from build123d import *

# Parameters (mm, degrees)
SKETCH2_R            = 3.9
BOSS_EXTRUDE1_DEPTH  = 12
SKETCH3_R            = 6
BOSS_EXTRUDE2_DEPTH  = 2
BOSS_EXTRUDE3_START  = 2
SKETCH4_R            = 6
BOSS_EXTRUDE3_DEPTH  = 2
SKETCH5_W            = 19.497175456
SKETCH5_H            = 13.883202756
CUT_EXTRUDE1_DEPTH   = 5
SKETCH6_W            = 2
SKETCH6_H            = 6.63324958
BOSS_EXTRUDE4_DEPTH  = 8
SKETCH7_W            = 16
SKETCH7_H            = 10
BOSS_EXTRUDE5_DEPTH  = 3
SKETCH8_R            = 12.5
BOSS_EXTRUDE6_DEPTH  = 40
SKETCH10_R           = 2.1
CUT_EXTRUDE2_DEPTH   = 21
BOSS_EXTRUDE7_DEPTH  = 12
FILLET1_R            = 0.5
SKETCH11_W           = 2
SKETCH11_H           = 19
BOSS_EXTRUDE8_DEPTH  = 11.3
SKETCH13_W           = 2
SKETCH13_H           = 19
BOSS_EXTRUDE9_DEPTH  = 11.3
SKETCH14_W           = 16
SKETCH14_H           = 19
BOSS_EXTRUDE10_DEPTH = 1
SKETCH15_W           = 16
SKETCH15_H           = 19
BOSS_EXTRUDE11_DEPTH = 1
SKETCH16_W           = 16
SKETCH16_H           = 7.233308129
CUT_EXTRUDE3_DEPTH   = 7
SKETCH17_W           = 16
SKETCH17_H           = 7.233308129
CUT_EXTRUDE4_DEPTH   = 7
SKETCH18_W           = 2
SKETCH18_H           = 1
BOSS_EXTRUDE12_DEPTH = 6.633249581
SKETCH19_W           = 2
SKETCH19_H           = 1
BOSS_EXTRUDE13_DEPTH = 6.633249581


with BuildPart() as part:
    # Sketch2 → Boss-Extrude1 (new body)
    with BuildSketch(Plane(origin=(0, 0, 0), x_dir=(0, 0, -1), z_dir=(1, 0, 0))):
        Circle(SKETCH2_R)
    extrude(amount=BOSS_EXTRUDE1_DEPTH)

    # Sketch3 → Boss-Extrude2 (add)
    with BuildSketch(Plane(origin=(12, 0, 0), x_dir=(0, 0, -1), z_dir=(1, 0, 0))):
        Circle(SKETCH3_R)
    extrude(amount=BOSS_EXTRUDE2_DEPTH)

    # Sketch4 → Boss-Extrude3 (add)
    with BuildSketch(Plane.ZY.offset(BOSS_EXTRUDE3_START)):
        with Locations(Location((0, 0, 0), (0, 0, 180))):
            Circle(SKETCH4_R)
    extrude(amount=-BOSS_EXTRUDE3_DEPTH)

    # Sketch5 → Cut-Extrude1 (cut)
    with BuildSketch(Plane(origin=(0, 5, 0), x_dir=(1, 0, 0), z_dir=(0, 1, 0))):
        with Locations((6.056898372, 0.369839418)):
            Rectangle(SKETCH5_W, SKETCH5_H)
    extrude(amount=CUT_EXTRUDE1_DEPTH, mode=Mode.SUBTRACT)

    # Sketch6 → Boss-Extrude4 (add)
    with BuildSketch(Plane(origin=(0, 5, 0), x_dir=(1, 0, 0), z_dir=(0, 1, 0))):
        with Locations((13, 0)):
            Rectangle(SKETCH6_W, SKETCH6_H)
        with Locations((-1, 0)):
            Rectangle(SKETCH6_W, SKETCH6_H)
    extrude(amount=BOSS_EXTRUDE4_DEPTH)

    # Sketch7 → Boss-Extrude5 (add)
    with BuildSketch(Plane(origin=(0, 13, 0), x_dir=(1, 0, 0), z_dir=(0, 1, 0))):
        with Locations((6, 0)):
            Rectangle(SKETCH7_W, SKETCH7_H)
    extrude(amount=BOSS_EXTRUDE5_DEPTH)

    # Sketch8 → Boss-Extrude6 (add)
    with BuildSketch(Plane(origin=(0, 16, 0), x_dir=(1, 0, 0), z_dir=(0, 1, 0))):
        with Locations(Location((6, 0, 0), (0, 0, 270))):
            Circle(SKETCH8_R)
    extrude(amount=BOSS_EXTRUDE6_DEPTH)

    # Sketch10 → Cut-Extrude2 (cut)
    with BuildSketch(Plane(origin=(0, 56, 0), x_dir=(1, 0, 0), z_dir=(0, 1, 0))):
        with Locations(Location((6, 0, 0), (0, 0, 270))):
            Circle(SKETCH10_R)
    extrude(amount=-CUT_EXTRUDE2_DEPTH, mode=Mode.SUBTRACT)

    # Sketch12 → Boss-Extrude7 (add)
    with BuildSketch(Plane.ZY.offset(-12)):
        Polygon((-3.2, 4.2), (3.2, 4.2), (5, 9.2), (5.36, 10.2), (-5.36, 10.2), (-5, 9.2), align=None)
    extrude(amount=BOSS_EXTRUDE7_DEPTH)

    # Fillet1
    fillet1_edges = [part.edges().sort_by_distance(p)[0] for p in [
        (6, 4.2, -3.2),
        (6, 4.2, 3.2),
        (6, 10.2, 5.36),
        (6, 10.2, -5.36),
    ]]
    fillet(fillet1_edges, radius=FILLET1_R)

    # Sketch11 → Boss-Extrude8 (add)
    with BuildSketch(Plane.XY.offset(3.31662479)):
        with Locations((13, 3.5)):
            Rectangle(SKETCH11_W, SKETCH11_H)
        with Locations((-1, 3.5)):
            Rectangle(SKETCH11_W, SKETCH11_H)
    extrude(amount=BOSS_EXTRUDE8_DEPTH)

    # Sketch13 → Boss-Extrude9 (add)
    with BuildSketch(Plane(origin=(0, 0, -3.31662479), x_dir=(-1, 0, 0), z_dir=(0, 0, -1))):
        with Locations((-13, 3.5)):
            Rectangle(SKETCH13_W, SKETCH13_H)
        with Locations((1, 3.5)):
            Rectangle(SKETCH13_W, SKETCH13_H)
    extrude(amount=BOSS_EXTRUDE9_DEPTH)

    # Sketch14 → Boss-Extrude10 (add)
    with BuildSketch(Plane.XY.offset(14.61662479)):
        with Locations((6, 3.5)):
            Rectangle(SKETCH14_W, SKETCH14_H)
    extrude(amount=BOSS_EXTRUDE10_DEPTH)

    # Sketch15 → Boss-Extrude11 (add)
    with BuildSketch(Plane(origin=(0, 0, -14.61662479), x_dir=(-1, 0, 0), z_dir=(0, 0, -1))):
        with Locations((-6, 3.5)):
            Rectangle(SKETCH15_W, SKETCH15_H)
    extrude(amount=BOSS_EXTRUDE11_DEPTH)

    # Sketch16 → Cut-Extrude3 (cut)
    with BuildSketch(Plane(origin=(0, 0, -15.61662479), x_dir=(-1, 0, 0), z_dir=(0, 0, -1))):
        with Locations((-6, 9.383345935)):
            Rectangle(SKETCH16_W, SKETCH16_H)
    extrude(amount=-CUT_EXTRUDE3_DEPTH, mode=Mode.SUBTRACT)

    # Sketch17 → Cut-Extrude4 (cut)
    with BuildSketch(Plane.XY.offset(15.61662479)):
        with Locations((6, 9.383345935)):
            Rectangle(SKETCH17_W, SKETCH17_H)
    extrude(amount=-CUT_EXTRUDE4_DEPTH, mode=Mode.SUBTRACT)

    # Sketch18 → Boss-Extrude12 (add)
    with BuildSketch(Plane(origin=(0, 0, 3.31662479), x_dir=(-1, 0, 0), z_dir=(0, 0, -1))):
        with Locations((-13, -5.5)):
            Rectangle(SKETCH18_W, SKETCH18_H)
    extrude(amount=BOSS_EXTRUDE12_DEPTH)

    # Sketch19 → Boss-Extrude13 (add)
    with BuildSketch(Plane(origin=(0, 0, 3.31662479), x_dir=(-1, 0, 0), z_dir=(0, 0, -1))):
        with Locations((1, -5.5)):
            Rectangle(SKETCH19_W, SKETCH19_H)
    extrude(amount=BOSS_EXTRUDE13_DEPTH)


solid = part.part
CAD build for the part. Positions are in the model's coordinates, mm. A direction names the side the tool comes from. Coordinates: 2 decimals unless noted, no trailing zeros. Order: outer loops, then holes, each group sorted by start corner. A loop starts at its lowest first (then second) coordinate and runs counter-clockwise, first axis right, second up. Notation, with made-up numbers: (85.25, -26.75) -> (136.25, -26.75) arc R16 cw to (136.25, -16.75) -> close; hole circle Ø10 at (87, 88). An arc over 180 degrees is marked (long way). Answer in a Markdown table with one row per item.
1) Drill centre lines: line 1 (X direction, y = 51.25, z = 0); line 2 (X direction, y = 12, z = -5); line 3 (Y direction, x = 10.5, z = 10). Where is each one in solid material? Low to high.
Check values:
| item | result |
|---|---|
| line 1 | -6.5 to 3.9, 8.1 to 18.5 |
| line 2 | -2 to 0, 12 to 14 |
| line 3 | 16 to 56 |
2) Which spindle directions (+Z, -Z, +X, -X, +Y, -Y) get a long thin tool onto all of the face, cutting with end or side? Do faces 4 (the face through (6, 14, -5)), 5 (the face through (6, 14, 5)), 6 (the face through (8.082, 45.647, -0.273)), 7 (the face through (6.08, 7, 4.21)). Say none if no direction does.
Check values:
| item | result |
|---|---|
| face 4 | -Z, +X, -X |
| face 5 | +Z, +X, -X |
| face 6 | +Y |
| face 7 | none |
3) Band-saw the part on D-D (z = 0). List the corners of the cut face in (x, y).
Check values:
| item | result |
|---|---|
| outline | (-6.5, 16) -> (-2, 16) -> (-2, -6) -> (0, -6) -> (0, -3.9) -> (12, -3.9) -> (12, -6) -> (14, -6) -> (14, 16) -> (18.5, 16) -> (18.5, 56) -> (8.1, 56) -> (8.1, 35) -> (3.9, 35) -> (3.9, 56) -> (-6.5, 56) -> close; hole (0, 3.9) -> (12, 3.9) -> (12, 4.2) -> (0, 4.2) -> close; hole (0, 10.2) -> (12, 10.2) -> (12, 13) -> (0, 13) -> close |
4) Flat gauge pins, fed straight in: P1, Ø6.5, axis at y = 3, z = 4, coming from the -X side; P2, Ø8, axis at y = 42, z = -6, coming from the -X side; P3, Ø8, axis at y = 49.5, z = -5, coming from the -X side. Where does each tip first touch, or does it go through?
Check values:
| item | result |
|---|---|
| P1 | x = -2 |
| P2 | x = -6.34 |
| P3 | x = -6.46 |
5) Band-saw the part on A-A (z = 10). List the corners of the cut face in (x, y), and give its area (3 significant figures).
Check values:
| item | result |
|---|---|
| outline | (-2, -6) -> (0, -6) -> (0, 5.77) -> (-2, 5.77) -> close; (-1.5, 16) -> (13.5, 16) -> (13.5, 56) -> (-1.5, 56) -> close; (12, -6) -> (14, -6) -> (14, 5.77) -> (12, 5.77) -> close |
| area | 647 mm2 |
6) Band-saw the part on B-B (x = 6). Give the number of separate pieces and of enclosed holes in the cut face, and give its area (3 significant figures).
Check values:
| item | result |
|---|---|
| separate pieces | 5 |
| enclosed holes | 0 |
| area | 1,060 mm2 |
7) Mould opens along X. For faces 1 (the face through (14, 2, 0)), 2 (the face through (6.084, 7.066, -4.232)), 3 (the face through (13, 13, -7)) say: pulls with the +X half, pulls with the -X half, needs draft (parallel to the pull), parting line crosses it, or undercut.
Check values:
| item | result |
|---|---|
| face 1 | pulls with the +X half |
| face 2 | undercut |
| face 3 | needs draft |
8) Band-saw the part on C-C (y = 0). List the corners of the cut face in (x, z), and give its area (3 significant figures).
Check values:
| item | result |
|---|---|
| outline | (-2, -15.62) -> (14, -15.62) -> (14, 15.62) -> (-2, 15.62) -> close; hole (0, -14.62) -> (12, -14.62) -> (12, -3.9) -> (0, -3.9) -> close; hole (0, 3.9) -> (12, 3.9) -> (12, 14.62) -> (0, 14.62) -> close |
| area | 243 mm2 |
